CAD build for the part. Positions are in the model's coordinates, mm. Face numbers are marked on the shaded views. A direction names the side the tool comes from. Coordinates: 2 decimals unless noted, no trailing zeros. Loops run counter-clockwise (first coordinate to the right, second up) from the corner with the lowest first, then second, coordinate; pieces in that order, holes last. Notation, with made-up numbers: (3.25, 13) - (54.25, 13) arc R18 ccw to (54.25, 19) - close; hole circle Ø11 at (59.5, 86.5). An arc over 180 degrees is marked (long way). Put each result on its own line as item: value.
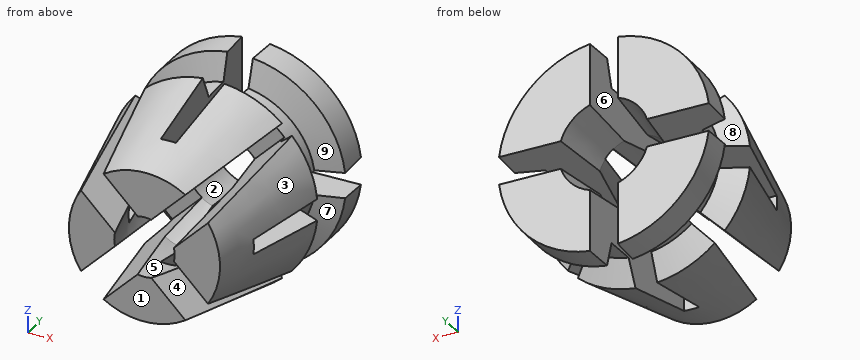
```python
from build123d import *

# Parameters (mm, degrees)
F3_DEPTH = 12.7
F4_COUNT = 2
F4_ANGLE = 90
F8_DEPTH = 12.7
F9_COUNT = 2
F9_ANGLE = 90


with BuildPart() as f1:
    # F0 (on Top) → F1 (revolve)
    with BuildSketch(Plane.XY):
        Polygon((7, 14), (3, 14), (2.5, 10), (3.275, 6), (2, 0), (5, 0), (6.889415849, 8.6733910541), (5.25, 9.4779638621), (5.25, 11.4779638621), (7, 12), align=None)
    revolve(axis=Axis((0, 3.7037534639, 0), (0, -1, 0)))


with BuildPart() as f3:
    # F2 (on Top) → F3 (new body, symmetric)
    with BuildSketch(Plane.XY):
        Polygon((0, 3), (0.5, 3), (1, 16), (0, 16), (-1, 16), (-0.5, 3), align=None)
    extrude(amount=F3_DEPTH, both=True)


with BuildPart() as f4_1:
    # F4: instance of F3
    add(f3.part.rotate(Axis((0, 3.7037534639, 0), (0, -1, 0)), 1 * F4_ANGLE / (F4_COUNT - 1)))


with BuildPart() as f1_1:
    add(f1.part)

    # F5: cut F3, F4_1
    add(f3.part, mode=Mode.SUBTRACT)
    add(f4_1.part, mode=Mode.SUBTRACT)


with BuildPart() as f8:
    # F7 (on line) → F8 (new body, symmetric)
    with BuildSketch(Plane(origin=(0, 0, 0), x_dir=(0.7071067812, 0, 0.7071067812), z_dir=(0.7071067812, 0, -0.7071067812))):
        Polygon((0.375, -10.0240074396), (1.125, 0.9756837906), (-1.125, 0.9756837906), (-0.375, -10.0240074396), align=None)
    extrude(amount=F8_DEPTH, both=True)


with BuildPart() as f9_1:
    # F9: instance of F8
    add(f8.part.rotate(Axis((0, 3.7037534639, 0), (0, -1, 0)), 1 * F9_ANGLE / (F9_COUNT - 1)))


with BuildPart() as f1_2:
    add(f1_1.part)

    # F10: cut F8, F9_1
    add(f8.part, mode=Mode.SUBTRACT)
    add(f9_1.part, mode=Mode.SUBTRACT)


solid = f1_2.part
```
Q1. Slice it at B-B, the plane y = 3.5. State how many separate pieces and enclosed holes the cut face has, then the cut area to 3 significant figures.
Determined:
separate pieces: 8
enclosed holes: 0
area: 48.2 mm2
Q2. Wall check: L1, parallel to X at y = 3.75, z = -3.25; L2, parallel to Z at x = 3, y = 2.75; L3, parallel to Z at x = -2, y = 1. Give the ranges that are in metal, low to high. Write a range as from..to.
Determined:
L1: -4.82..-4.39, -2.11..-0.53, 0.53..2.11, 4.39..4.82
L2: -4.73..-4.23, -1.77..1.77, 4.23..4.73
L3: -4.82..-3.4, 3.4..4.82
Q3. Slice it at A-A, the plane y = 1.25. Give the cut face in (x, z).
Determined:
outline: (-4.35, -2.98) - (-2.13, -0.76) arc R2.27 cw to (-2.13, 0.76) - (-4.35, 2.98) arc R5.27 ccw to start; (-2.98, -4.35) arc R5.27 ccw to (2.98, -4.35) - (0.76, -2.13) arc R2.27 cw to (-0.76, -2.13) - close; (-2.98, 4.35) - (-0.76, 2.13) arc R2.27 cw to (0.76, 2.13) - (2.98, 4.35) arc R5.27 ccw to start; (2.13, -0.76) - (4.35, -2.98) arc R5.27 ccw to (4.35, 2.98) - (2.13, 0.76) arc R2.27 cw to start
Q4. Mould opens along Z. For the marked faces 1, 2, 3 and 4 say: +Z half, -Z half, draft (parallel to the pull), parting line (faces both ways), or undercut.
Determined:
face 1: draft
face 2: undercut
face 3: parting line
face 4: undercut
Q5. Tool access for the marked faces 5, 6, 7, 8 and 9: list every direction of +Z, -Z, +X, -X, +Y, -Y with a clear straight run to the whole face (end or side of a thin tool).
Determined:
face 5: none
face 6: +Z, -Z, +Y
face 7: -Z, +X
face 8: +Z, -X
face 9: +Z, +X
Q6. Pin check, flat tips, straight feed: pin 1 Ø0.8 at (x, z) = (0, 4) entering from +Y; pin 2 Ø1.5 at (x, y) = (-5, 9.5) entering from -Z; pin 3 Ø1 at (y, z) = (1.5, 4) entering from -X. Stop position of each tip, or through.
Determined:
pin 1: y = 3
pin 2: z = -4.42
pin 3: x = -3.09
